Read the model definition and answer for the solid it produces. Units are mm, in the model's axes. A direction names the side the tool comes from. Coordinates: 2 decimals unless noted, no trailing zeros. Order: outer loops, then holes, each group sorted by start corner. A loop starts at its lowest first (then second) coordinate and runs counter-clockwise, first axis right, second up. Notation, with made-up numbers: M 60,73 L 102,73 A21 ccw 102,111 Z; hole C -10,59.25 d6. An arc over 180 degrees is marked long. Use a Markdown table: item, result. Add a question column.
1) Find section A-A on z = 7.25. Write down the section's boundary in (x, y), plus the area to 3 significant figures.
2) For faces 1 (the face through (-10.107, 12, 4)), 2 (the face through (16, 5.581, 4)), 3 (the face through (0, 12, 9)), determine the directions among +Z, -Z, +X, -X, +Y, -Y from which every point of the face is accessible in a straight line to the end or side of a thin tool.
3) Find the intervals of material crossed by probe 1 along Y at (x, z) = (-13, 6); probe 2 along Y at (x, z) = (-17, 8.75); probe 3 along Z at (x, y) = (-12.5, 9), in increasing order. Write a range as [from, to].
4) Find section C-C on x = -17. Write down the section's boundary in (y, z), plus the area to 3 significant figures.
5) The mould has two halves that part along Y. Classify faces 4 (the face through (0.431, 9.724, 4.563)), 5 (the face through (0, -3.119, 4)), 6 (the face through (22.893, 6, 1)): released by +Y, released by -Y, zero draft, split by the parting line, or undercut.
6) Each of these flat-tipped pins is pushed along its axis until it touches: pin 1 Ø2 at (y, z) = (15.5, 4.5) entering from -X; pin 2 Ø1.5 at (x, y) = (-11.5, 11) entering from -Z; pin 3 Ø11.5 at (x, y) = (-18.5, 7) entering from +Z; pin 4 Ø3.5 at (y, z) = (14, 5) entering from +X. Where does it stop, or does it pass through?
7) Find section D-D on z = 4.25. Write down the section's boundary in (x, y), plus the area to 3 significant figures.
8) Find section B-B on y = 14.5. Write down the section's boundary in (x, z).
from build123d import *

# Parameters (mm, degrees)
ESQUISSE1_W             = 46
ESQUISSE1_H             = 24
BOSS_EXTRU_1_DEPTH      = 9
ESQUISSE2_R             = 1
ENL_V_MAT_EXTRU_1_DEPTH = 19
ESQUISSE3_W             = 15.6
ESQUISSE3_H             = 21.4
ENL_V_MAT_EXTRU_2_DEPTH = 2.4
ESQUISSE4_W             = 14
ESQUISSE4_H             = 13
ENL_V_MAT_EXTRU_3_DEPTH = 4.5


with BuildPart() as part:
    # Esquisse1 → Boss.-Extru.1 (new body)
    with BuildSketch(Plane.XY):
        with Locations((-0.106918239, 8.880503145)):
            Rectangle(ESQUISSE1_W, ESQUISSE1_H)
    extrude(amount=BOSS_EXTRU_1_DEPTH)

    # Esquisse2 → Enlèv. mat.-Extru.1 (cut)
    with BuildSketch(Plane.XY.offset(9)):
        with Locations((-0.106918239, 8.880503145)):
            Circle(ESQUISSE2_R)
    extrude(amount=-ENL_V_MAT_EXTRU_1_DEPTH, mode=Mode.SUBTRACT)

    # Esquisse3 → Enlèv. mat.-Extru.2 (cut)
    with BuildSketch(Plane.XY.offset(9)):
        with Locations((-16.406918239, 8.880503145)):
            Rectangle(ESQUISSE3_W, ESQUISSE3_H)
        with Locations((16.193081761, 8.880503145)):
            Rectangle(ESQUISSE3_W, ESQUISSE3_H)
    extrude(amount=-ENL_V_MAT_EXTRU_2_DEPTH, mode=Mode.SUBTRACT)

    # Esquisse4 → Enlèv. mat.-Extru.3 (cut)
    with BuildSketch(Plane.XY.offset(6.6)):
        with Locations((-17.106918239, 12.080503145)):
            Rectangle(ESQUISSE4_W, ESQUISSE4_H)
        with Locations((16.893081761, 12.080503145)):
            Rectangle(ESQUISSE4_W, ESQUISSE4_H)
    extrude(amount=-ENL_V_MAT_EXTRU_3_DEPTH, mode=Mode.SUBTRACT)


solid = part.part
Check result:
| question | item | result |
|---|---|---|
| 1 | outline | M -23.11,-3.12 L 22.89,-3.12 L 22.89,-1.82 L 8.39,-1.82 L 8.39,19.58 L 22.89,19.58 L 22.89,20.88 L -23.11,20.88 L -23.11,19.58 L -8.61,19.58 L -8.61,-1.82 L -23.11,-1.82 Z; hole C -0.11,8.88 d2 |
| 1 | area | 480 mm2 |
| 2 | face 1 | +Z, -X |
| 2 | face 2 | +Z, +X |
| 2 | face 3 | +Z, +X, -X, +Y, -Y |
| 3 | probe 1 | y = [-3.12, 5.58], [18.58, 20.88] |
| 3 | probe 2 | y = [-3.12, -1.82], [19.58, 20.88] |
| 3 | probe 3 | z = [0, 2.1] |
| 4 | outline | M -3.12,0 L 20.88,0 L 20.88,9 L 19.58,9 L 19.58,6.6 L 18.58,6.6 L 18.58,2.1 L 5.58,2.1 L 5.58,6.6 L -1.82,6.6 L -1.82,9 L -3.12,9 Z |
| 4 | area | 106 mm2 |
| 5 | face 4 | undercut |
| 5 | face 5 | released by -Y |
| 5 | face 6 | zero draft |
| 6 | pin 1 | stops at x = -10.11 |
| 6 | pin 2 | stops at z = 0 |
| 6 | pin 3 | stops at z = 6.6 |
| 6 | pin 4 | stops at x = 9.89 |
| 7 | outline | M -23.11,-3.12 L 22.89,-3.12 L 22.89,5.58 L 9.89,5.58 L 9.89,18.58 L 22.89,18.58 L 22.89,20.88 L -23.11,20.88 L -23.11,18.58 L -10.11,18.58 L -10.11,5.58 L -23.11,5.58 Z; hole C -0.11,8.88 d2 |
| 7 | area | 763 mm2 |
| 8 | outline | M -23.11,0 L 22.89,0 L 22.89,2.1 L 9.89,2.1 L 9.89,6.6 L 8.39,6.6 L 8.39,9 L -8.61,9 L -8.61,6.6 L -10.11,6.6 L -10.11,2.1 L -23.11,2.1 Z |
